For this review, use the dimensioned drawing (mm, ordinates from the lowest corner) and the shaded views. A direction names the side the tool comes from. Coordinates: 2 decimals unless noted, no trailing zeros. Order: outer loops, then holes, each group sorted by start corner. A loop starts at its lowest first (then second) coordinate and runs counter-clockwise, first axis right, second up. Notation, with made-up numbers: M -23.75,82 L 26.25,82 A22 ccw 26.25,88 Z; hole C -21,19.25 d8. An arc over 180 degrees is marked long. One line per item, written item: value.
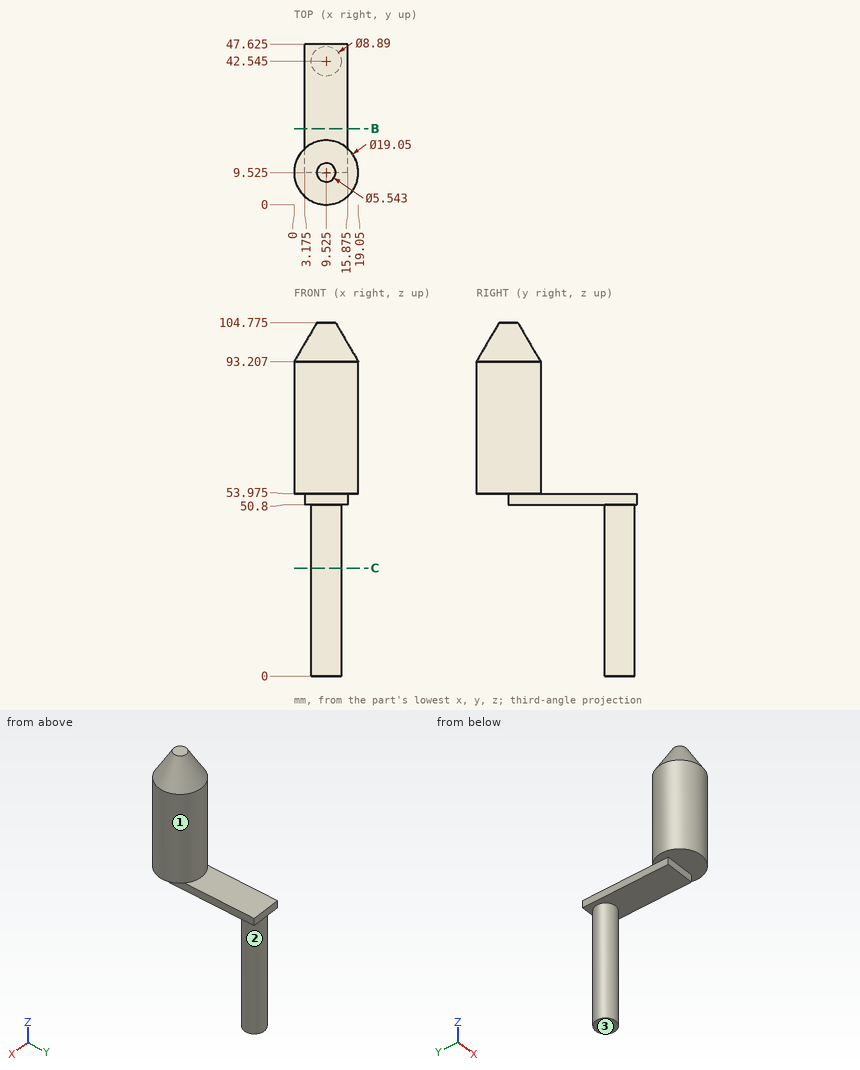
(1) For L1, parallel to Z at x = 4, y = 38.5 (1 decimal); L2, parallel to Z at x = 12.5, y = 40 (1 decimal); L3, parallel to Y at x = 9.5, z = 39.5, list the stretches that pass through material, from the lowest coordinate up.
Geometry results:
L1: z = 50.8 to 54
L2: z = 0 to 54
L3: y = 38.1 to 46.99
(2) Tool access review of the marked faces 1, 2 and 3: name each direction out of +Z, -Z, +X, -X, +Y, -Y from which nothing blocks a thin tool from reaching the whole face with its end or side.
Geometry results:
face 1: +Z
face 2: -Z
face 3: -Z, +X, -X, +Y, -Y
(3) We need section B-B, the plane y = 22.5. State the section outline as (x, z) points (1 decimal), plus the area to 3 significant figures.
Geometry results:
outline: M 3.2,50.8 L 15.9,50.8 L 15.9,54 L 3.2,54 Z
area: 40.3 mm2
(4) Insertion check: pin 1 Ø4 at (x, z) = (15, 16.5) entering from -Y; pin 2 Ø6.5 at (x, y) = (9.5, 30) entering from -Z; pin 3 Ø3.5 at (y, z) = (37, 53) entering from +X (3 decimals). Each pin has a flat end and moves straight along its axis. Give the tip position at first contact, or say it passes through.
Geometry results:
pin 1: stops at y = 39.77
pin 2: stops at z = 50.8
pin 3: stops at x = 15.875
(5) We need section C-C, the plane z = 32. State the section outline as (x, y) points (1 decimal), plus the area to 3 significant figures.
Geometry results:
outline: C 9.5,42.5 d8.9
area: 62.1 mm2
